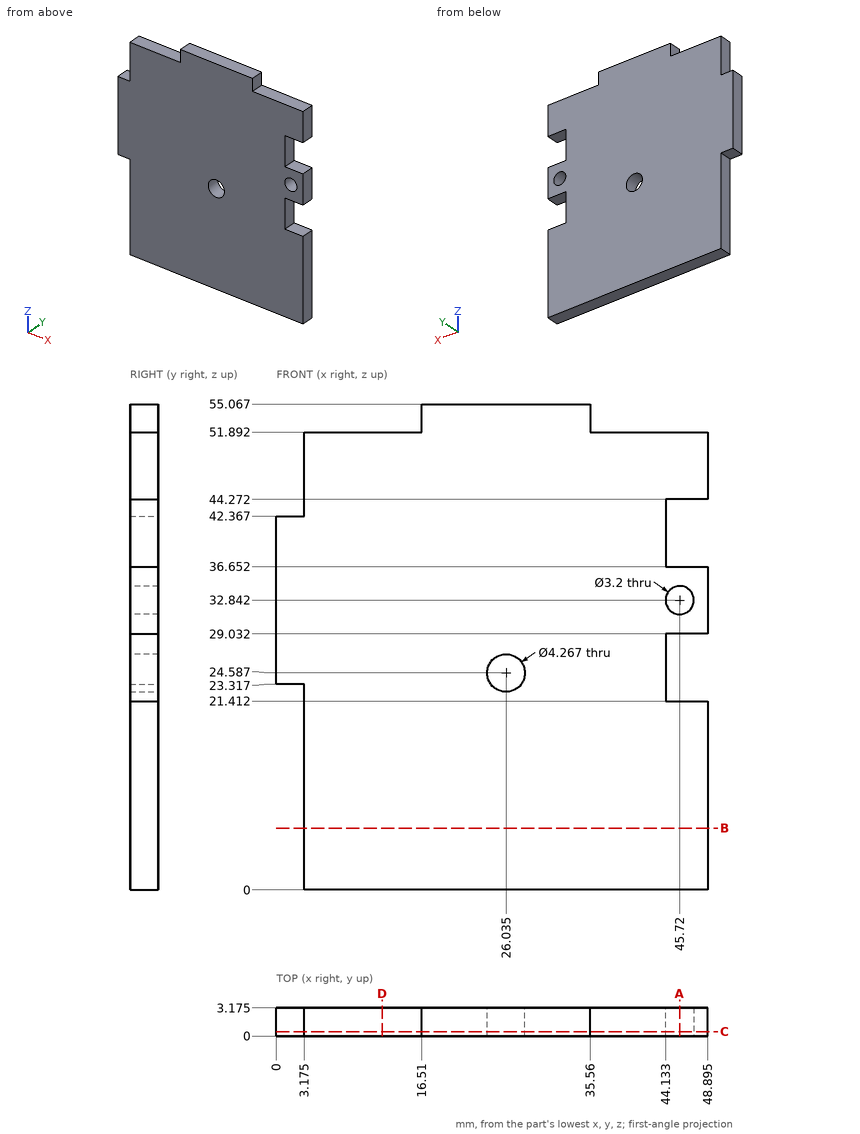
Can you work these out from the drawing? Everything is in mm from the part's minimum corner. Round coordinates to 2 decimals unless told otherwise and drop trailing zeros. Loops run counter-clockwise (first coordinate to the right, second up) from the corner with the lowest first, then second, coordinate; pieces in that order, holes last. Notation, with made-up numbers: (-40, 59.5) - (19, 59.5) arc R27 ccw to (19, 98.5) - close; hole circle Ø8 at (10.5, -33.5). An arc over 180 degrees is marked (long way). Answer in a Markdown table with one row per item. Add a question column.
(1) I need wall thicknesses on line 1 along Z through (x, y) = (15, 1.75); line 2 along X through (y, z) = (1.9, 12) (1 decimal); line 3 along X through (y, z) = (2.2, 22) (1 decimal). Which ranges of each line are inside material? Lowest first, please.
(2) If we section it at D-D (x = 12): Please give me the cut outline in (y, z) (1 decimal).
(3) If we section it at A-A (x = 45.72): Please give me the cut outline in (y, z) (1 decimal).
(4) If we section it at B-B (z = 7): Please give me the cut outline in (x, y) (1 decimal).
(5) I'm going to push flat-ended pins straight in: pin 1 (1 mm diameter, centred on x = 47, y = 1.5, fed in from +Z); pin 2 (1 mm diameter, centred on y = 1, z = 53, fed in from +X); pin 3 (1.6 mm diameter, centred on y = 2, z = 53.5, fed in from -X). Where does each tip first touch, or does it pass through?
(6) If we section it at C-C (y = 0.5): Please give me the cut outline in (x, z) (1 decimal), plus the area to 3 significant figures.
Model answer:
| question | item | result |
|---|---|---|
| 1 | line 1 | z = 0 to 51.89 |
| 1 | line 2 | x = 3.2 to 48.9 |
| 1 | line 3 | x = 3.2 to 44.1 |
| 2 | outline | (0, 0) - (3.2, 0) - (3.2, 51.9) - (0, 51.9) - close |
| 3 | outline | (0, 0) - (3.2, 0) - (3.2, 21.4) - (0, 21.4) - close; (0, 29) - (3.2, 29) - (3.2, 31.2) - (0, 31.2) - close; (0, 34.4) - (3.2, 34.4) - (3.2, 36.7) - (0, 36.7) - close; (0, 44.3) - (3.2, 44.3) - (3.2, 51.9) - (0, 51.9) - close |
| 4 | outline | (3.2, 0) - (48.9, 0) - (48.9, 3.2) - (3.2, 3.2) - close |
| 5 | pin 1 | stops at z = 51.89 |
| 5 | pin 2 | stops at x = 35.56 |
| 5 | pin 3 | stops at x = 16.51 |
| 6 | outline | (0, 23.3) - (3.2, 23.3) - (3.2, 0) - (48.9, 0) - (48.9, 21.4) - (44.1, 21.4) - (44.1, 29) - (48.9, 29) - (48.9, 36.7) - (44.1, 36.7) - (44.1, 44.3) - (48.9, 44.3) - (48.9, 51.9) - (35.6, 51.9) - (35.6, 55.1) - (16.5, 55.1) - (16.5, 51.9) - (3.2, 51.9) - (3.2, 42.4) - (0, 42.4) - close; hole circle Ø4.3 at (26, 24.6); hole circle Ø3.2 at (45.7, 32.8) |
| 6 | area | 2,400 mm² |
